from build123d import *

# Parameters (mm, degrees)
BOSS_EXTRUDE2_DEPTH = 96
SKETCH2_W           = 418
SKETCH2_H           = 194
BOSS_EXTRUDE3_DEPTH = 10
SKETCH3_R           = 20
BOSS_EXTRUDE5_DEPTH = 15
SKETCH3_4_W         = 15.513986376
SKETCH3_4_H         = 16.487812262
SKETCH3_4_W_2       = 16.085927628
SKETCH3_4_H_2       = 15.566266702
BOSS_EXTRUDE6_DEPTH = 25
SKETCH3_6_R         = 20
BOSS_EXTRUDE7_DEPTH = 15
SKETCH4_W           = 85.572953824
SKETCH4_H           = 51.067730508
BOSS_EXTRUDE8_DEPTH = 15


with BuildPart() as part:
    # Sketch1 → Boss-Extrude2 (new body)
    with BuildSketch(Plane(origin=(0, 0, 0), x_dir=(1, 0, 0), z_dir=(0, 1, 0))):
        with BuildLine():
            Line((-209, -60.2), (-209, -87))
            ThreePointArc((-209, -87), (-206.071067812, -94.071067812), (-199, -97))
            Line((-199, -97), (0, -97))
            Line((0, -97), (0, 97))
            Line((0, 97), (-199, 97))
            ThreePointArc((-199, 97), (-206.071067812, 94.071067812), (-209, 87))
            Line((-209, 87), (-209, 61.169229263))
            Line((-209, 61.169229263), (-209, 56.20183264))
            Line((-209, 56.20183264), (-198.157814389, 56.20183264))
            ThreePointArc((-198.157814389, 56.20183264), (-191.086746578, 53.272900452), (-188.157814389, 46.20183264))
            Line((-188.157814389, 46.20183264), (-188.157814389, -50.2))
            ThreePointArc((-188.157814389, -50.2), (-191.086746578, -57.271067812), (-198.157814389, -60.2))
            Line((-198.157814389, -60.2), (-209, -60.2))
        make_face()
        with BuildLine():
            Line((0, 97), (0, -97))
            Line((0, -97), (199, -97))
            ThreePointArc((199, -97), (206.071067812, -94.071067812), (209, -87))
            Line((209, -87), (209, -60.2))
            Line((209, -60.2), (198.157814389, -60.2))
            ThreePointArc((198.157814389, -60.2), (191.086746578, -57.271067812), (188.157814389, -50.2))
            Line((188.157814389, -50.2), (188.157814389, 46.20183264))
            ThreePointArc((188.157814389, 46.20183264), (191.086746578, 53.272900452), (198.157814389, 56.20183264))
            Line((198.157814389, 56.20183264), (209, 56.20183264))
            Line((209, 56.20183264), (209, 87))
            ThreePointArc((209, 87), (206.071067812, 94.071067812), (199, 97))
            Line((199, 97), (0, 97))
        make_face()
    extrude(amount=BOSS_EXTRUDE2_DEPTH)

    # Sketch2 → Boss-Extrude3 (add)
    with BuildSketch(Plane(origin=(0, 96, 0), x_dir=(1, 0, 0), z_dir=(0, 1, 0))):
        Rectangle(SKETCH2_W, SKETCH2_H)
    extrude(amount=BOSS_EXTRUDE3_DEPTH)

    # Sketch3 → Boss-Extrude5 (add)
    with BuildSketch(Plane(origin=(0, 96, 0), x_dir=(1, 0, 0), z_dir=(0, 1, 0))):
        with Locations(Location((-104.5, 48.5, 0), (0, 0, 90))):
            Circle(SKETCH3_R)
    extrude(amount=BOSS_EXTRUDE5_DEPTH)

    # Sketch3_4 → Boss-Extrude6 (add)
    with BuildSketch(Plane(origin=(0, 96, 0), x_dir=(1, 0, 0), z_dir=(0, 1, 0))):
        with Locations((-104.5, 48.5)):
            Rectangle(SKETCH3_4_W, SKETCH3_4_H)
        with Locations((104.5, -48.5)):
            Rectangle(SKETCH3_4_W_2, SKETCH3_4_H_2)
    extrude(amount=BOSS_EXTRUDE6_DEPTH)

    # Sketch3_6 → Boss-Extrude7 (add)
    with BuildSketch(Plane(origin=(0, 96, 0), x_dir=(1, 0, 0), z_dir=(0, 1, 0))):
        with Locations(Location((104.5, -48.5, 0), (0, 0, 90))):
            Circle(SKETCH3_6_R)
    extrude(amount=BOSS_EXTRUDE7_DEPTH)

    # Sketch4 → Boss-Extrude8 (add)
    with BuildSketch(Plane(origin=(0, 96, 0), x_dir=(1, 0, 0), z_dir=(0, 1, 0))):
        Rectangle(SKETCH4_W, SKETCH4_H)
    extrude(amount=BOSS_EXTRUDE8_DEPTH)


solid = part.part
The listing builds one solid part. Answer for the finished solid, in the listing's coordinates (mm). A direction names the side the tool comes from. Give positions to 0.01 mm unless a question says otherwise; leave off trailing zeros. Order: outer loops, then holes, each group sorted by start corner. A loop starts at its lowest first (then second) coordinate and runs counter-clockwise, first axis right, second up. Notation, with made-up numbers: (-38, 45.5) - (-11, 45.5) arc R23 cw to (-11, 74.5) - close; hole circle Ø6 at (72.5, -18.75). An arc over 180 degrees is marked (long way). One line per item, written item: value. Start each with the question number.
1) A tool of negligible diameter and unlimited length cuts with its end or side. For faces 4 (the face through (-191.009, 47.328, 57.193)), 5 (the face through (122.243, 108.465, 39.271)), 6 (the face through (-105, 116, -56.744)), from which of +Z, -Z, +X, -X, +Y, -Y can it reach the whole face along a straight path? Write none if from no direction.
2) The mould has two halves that part along Z. Classify faces 1 (the face through (112.543, 116, 49)), 2 (the face through (-199, 96, 1)), 3 (the face through (-3, 52, -97)): released by +Z, released by -Z, zero draft, split by the parting line, or undercut.
3) Given pin 1 Ø2 at (y, z) = (63.5, 26) entering from -X; pin 2 Ø1 at (y, z) = (62.5, 3.5) entering from +X; pin 3 Ø4 at (y, z) = (109, 12.5) entering from -X, each flat-ended and moving along its own axis, determine where each tip first touches the part or whether it passes through.
4) A cutting plane is placed at A-A on x = 104.5. Give the vertices of the cut face in (y, z), then the cut area to 3 significant figures.
5) A cutting plane is placed at C-C on x = -104.5. Give the vertices of the cut face in (y, z), then the cut area to 3 significant figures.
6) A cutting plane is placed at B-B on y = 71. Give the vertices of the cut face in (x, z).
7) Find the intervals of material crossed by L1, parallel to Y at x = 4, z = 43.5; L2, parallel to Y at x = -190.5, z = -50; L3, parallel to X at y = 16, z = -17, in increasing order.
Answer sheet:
1. face 4: -X, -Y
1. face 5: +Y
1. face 6: -Z, +X, -X, +Y
2. face 1: zero draft
2. face 2: undercut
2. face 3: released by -Z
3. pin 1: stops at x = -188.16
3. pin 2: stops at x = 188.16
3. pin 3: stops at x = -42.79
4. outline: (0, -97) - (106, -97) - (106, 28.5) - (111, 28.5) - (111, 40.72) - (121, 40.72) - (121, 56.28) - (111, 56.28) - (111, 68.5) - (106, 68.5) - (106, 97) - (0, 97) - close
4. area: 20,900 mm2
5. outline: (0, -97) - (106, -97) - (106, -68.5) - (111, -68.5) - (111, -56.74) - (121, -56.74) - (121, -40.26) - (111, -40.26) - (111, -28.5) - (106, -28.5) - (106, 97) - (0, 97) - close
5. area: 20,900 mm2
6. outline: (-209, -87) arc R10 ccw to (-199, -97) - (199, -97) arc R10 ccw to (209, -87) - (209, -56.2) - (198.16, -56.2) arc R10 cw to (188.16, -46.2) - (188.16, 50.2) arc R10 cw to (198.16, 60.2) - (209, 60.2) - (209, 87) arc R10 ccw to (199, 97) - (-199, 97) arc R10 ccw to (-209, 87) - (-209, 60.2) - (-198.16, 60.2) arc R10 cw to (-188.16, 50.2) - (-188.16, -46.2) arc R10 cw to (-198.16, -56.2) - (-209, -56.2) - close
7. L1: y = 0 to 106
7. L2: y = 96 to 106
7. L3: x = -188.16 to 188.16
